Autodesk Inventor part; units mm, degrees
ref_plane "YZ Plane" through (0, 0, 0) normal (1, 0, 0) x (0, 1, 0)
ref_plane "XZ Plane" through (0, 0, 0) normal (0, 1, 0) x (-1, 0, 0)
ref_plane "XY Plane" through (0, 0, 0) normal (0, 0, 1) x (1, 0, 0)
sketch "Sketch1" plane through (0, 0, 0) normal (0, 0, 1) x (1, 0, 0)
  line L0 (0, 0) -> (55.5, 0)
  line L1 (55.5, 0) -> (55.5, 32.4)
  line L2 (55.5, 32.4) -> (0, 32.4)
  line L3 (0, 32.4) -> (0, 0)
  circle A0 centre (3.5, 28.9) radius 1.5
  circle A1 centre (52, 28.9) radius 1.5
  circle A2 centre (3.5, 3.5) radius 1.5
  circle A3 centre (52, 3.5) radius 1.5
  dimension "d0" = 55.5
  dimension "d1" = 32.4
  dimension "d2" = 3
  dimension "d3" = 3
  dimension "d4" = 3
  dimension "d5" = 3
  dimension "d6" = 3.5
  dimension "d7" = 3.5
  dimension "d8" = 3.5
  dimension "d9" = 3.5
  dimension "d10" = 3.5
  dimension "d11" = 3.5
  dimension "d12" = 3.5
  dimension "d13" = 3.5
extrude "Extrusion1" add sketch "Sketch1" along normal blind 1.6
fillet "Fillet1" radius 4 4 edges at (55.5, 32.4, 0.8) (55.5, 0, 0.8) (0, 0, 0.8) (0, 32.4, 0.8)
sketch "Sketch2" plane through (0, 0, 1.6) normal (0, 0, 1) x (1, 0, 0)
  circle A0 centre (15.6251, 23.6367) radius 4.3835
  circle A1 centre (39.6101, 23.6367) radius 5.1943
  line L0 (1.8909, 21.1486) -> (6.469, 21.1486)
  line L1 (6.469, 21.1486) -> (6.469, 11.893)
  line L2 (6.469, 11.893) -> (1.8909, 11.893)
  line L3 (1.8909, 11.893) -> (1.8909, 21.1486)
  line L4 (48.8658, 21.1486) -> (53.8419, 21.1486)
  line L5 (53.8419, 21.1486) -> (53.8419, 11.893)
  line L6 (53.8419, 11.893) -> (48.8658, 11.893)
  line L7 (48.8658, 11.893) -> (48.8658, 21.1486)
  line L8 (21.0989, 30.2052) -> (31.4492, 30.2052)
  line L9 (31.4492, 30.2052) -> (31.4492, 19.8548)
  line L10 (31.4492, 19.8548) -> (21.0989, 19.8548)
  line L11 (21.0989, 19.8548) -> (21.0989, 30.2052)
  line L12 (18.7103, 13.4854) -> (22.9898, 13.4854)
  line L13 (22.9898, 13.4854) -> (22.9898, 2.9359)
  line L14 (22.9898, 2.9359) -> (18.7103, 2.9359)
  line L15 (18.7103, 2.9359) -> (18.7103, 13.4854)
  point P0 (0, 0)
extrude "Extrusion2" add sketch "Sketch2" along normal blind 10.7
sketch "Sketch3" plane through (0, 0, 12.3) normal (0, 0, 1) x (1, 0, 0)
  circle A0 centre (19.5755, 4.3447) radius 0.7457
  point P0 (0, 0)
extrude "Extrusion3" add sketch "Sketch3" along normal blind 1.18
properties part number "PowerSupply"
Geometry check sheet. Reference: the model listing, model coordinates, mm. A direction names the side the tool comes from. Give positions to 0.01 mm unless a question says otherwise; leave off trailing zeros. Loops run counter-clockwise (first coordinate to the right, second up) from the corner with the lowest first, then second, coordinate; pieces in that order, holes last. Notation, with made-up numbers: M 10,23 L 39,23 A8 cw 39,27 Z; hole C 77,26 d3. An arc over 180 degrees is marked long. Write item = value, one per line.
(1) Sectioned sample at B-B, the plane y = 6. Record the cut outline in (x, z).
Answer below:
outline = M 0,0 L 55.5,0 L 55.5,1.6 L 22.99,1.6 L 22.99,12.3 L 18.71,12.3 L 18.71,1.6 L 0,1.6 Z
(2) Sectioned sample at A-A, the plane x = 26. Record the cut outline in (y, z), plus the area to 3 significant figures.
Answer below:
outline = M 0,0 L 32.4,0 L 32.4,1.6 L 30.21,1.6 L 30.21,12.3 L 19.85,12.3 L 19.85,1.6 L 0,1.6 Z
area = 163 mm2
(3) Material ranges on line 1 (X direction, y = 12.5, z = 5.5); line 2 (X direction, y = 23.5, z = 9.75); line 3 (X direction, y = 14.5, z = 10), recorded low to high. Write a range as [from, to].
Answer below:
line_1 = [1.89, 6.47], [18.71, 22.99], [48.87, 53.84]
line_2 = [11.24, 20.01], [21.1, 31.45], [34.42, 44.8]
line_3 = [1.89, 6.47], [48.87, 53.84]
(4) Gauge pin test, flat ends, axial feed: pin 1 Ø7 at (x, y) = (17, 24.5) entering from +Z; pin 2 Ø3 at (x, z) = (14.5, 11) entering from -Y; pin 3 Ø6 at (x, z) = (35.5, 11.5) entering from -Y. Record the tip position at first contact, or that the pin passes through.
Answer below:
pin_1 = 12.3
pin_2 = 19.25
pin_3 = 18.56
(5) Sectioned sample at C-C, the plane z = 11.5. Record the cut outline in (x, y).
Answer below:
outline = M 1.89,11.89 L 6.47,11.89 L 6.47,21.15 L 1.89,21.15 Z; C 15.63,23.64 d8.77; M 18.71,2.94 L 22.99,2.94 L 22.99,13.49 L 18.71,13.49 Z; M 21.1,19.85 L 31.45,19.85 L 31.45,30.21 L 21.1,30.21 Z; C 39.61,23.64 d10.39; M 48.87,11.89 L 53.84,11.89 L 53.84,21.15 L 48.87,21.15 Z
(6) Sectioned sample at D-D, the plane y = 22.5. Record the cut outline in (x, z).
Answer below:
outline = M 0,0 L 55.5,0 L 55.5,1.6 L 44.68,1.6 L 44.68,12.3 L 34.54,12.3 L 34.54,1.6 L 31.45,1.6 L 31.45,12.3 L 21.1,12.3 L 21.1,1.6 L 19.86,1.6 L 19.86,12.3 L 11.39,12.3 L 11.39,1.6 L 0,1.6 Z
(7) Tool access check on faces 4 (the face through (1.891, 16, 7)), 5 (the face through (26, 30.205, 7)), 6 (the face through (26, 19.855, 7)), 7 (the face through (6.469, 17, 7)). Record the directions out of +Z, -Z, +X, -X, +Y, -Y that give a thin tool (end or side, any length) a straight path to the whole face; none if there is none.
Answer below:
face_4 = +Z, -X, +Y, -Y
face_5 = +Z, +X, -X, +Y
face_6 = +Z
face_7 = +Z, +Y, -Y
(8) Release check for a two-part mould opening along Y. For faces 1 (the face through (50.8, 4.4, 0.8)), 2 (the face through (1.141, 1.203, 0.811)), 3 (the face through (21, 8, 12.3)) record: released by +Y, released by -Y, zero draft, split by the parting line, or undercut.
Answer below:
face_1 = undercut
face_2 = released by -Y
face_3 = zero draft
